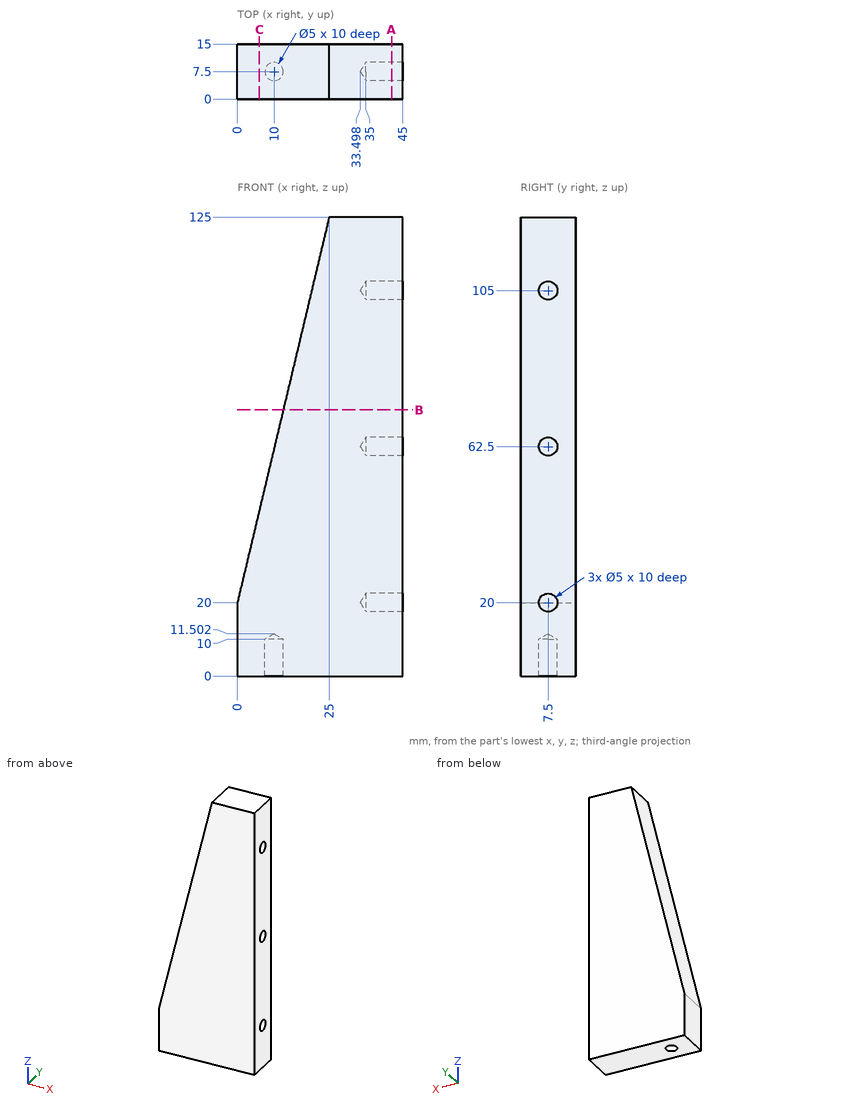
Could you check a few things on this drawing? It's one solid part, dimensions in mm from its lowest x, y, z. Give positions to 0.01 mm unless a question says otherwise; leave off trailing zeros. Order: outer loops, then holes, each group sorted by start corner. A loop starts at its lowest first (then second) coordinate and runs counter-clockwise, first axis right, second up. Notation, with made-up numbers: (-33.75, 51) - (-23.75, 51) arc R22 ccw to (-23.75, 79) - close; hole circle Ø4 at (18.25, 52.25). An arc over 180 degrees is marked (long way). Return JSON: item names as keys, results as strings. Group by question number.
Q1. Suppose I cut it at C-C, the plane x = 6. Please give me the cut outline in (y, z).
Q2. Suppose I cut it at B-B, the plane z = 72.5. Please give me the cut outline in (x, y), and give its area (4 significant figures).
Q3. Please list where these lines run through material, in increasing order: line 1 along Z through (x, y) = (40, 7.5); line 2 along Y through (x, z) = (39, 105); line 3 along X through (y, z) = (7.5, 7.5). Write a range as [from, to].
Q4. Suppose I cut it at A-A, the plane x = 42. Please give me the cut outline in (y, z), and give its area (3 significant figures).
Q5. Will these pins go through, and if not, where does the flat tip stop? pin 1 Ø1 at (y, z) = (13, 46.5) entering from -X; pin 2 Ø5 at (y, z) = (5.5, 92.5) entering from -X; pin 3 Ø3 at (y, z) = (7.5, 62.5) entering from +X.
Resolved:
{
 "1": {"outline": "(0, 0) - (15, 0) - (15, 45.2) - (0, 45.2) - close"},
 "2": {"outline": "(12.5, 0) - (45, 0) - (45, 15) - (12.5, 15) - close", "area": "487.5 mm2"},
 "3": {"line 1": "z = [0, 17.5], [22.5, 60], [65, 102.5], [107.5, 125]", "line 2": "y = [0, 5], [10, 15]", "line 3": "x = [0, 7.5], [12.5, 45]"},
 "4": {"outline": "(0, 0) - (15, 0) - (15, 125) - (0, 125) - close; hole circle Ø5 at (7.5, 20); hole circle Ø5 at (7.5, 62.5); hole circle Ø5 at (7.5, 105)", "area": "1,820 mm2"},
 "5": {"pin 1": "stops at x = 6.19", "pin 2": "stops at x = 16.67", "pin 3": "stops at x = 34.4"}
}
